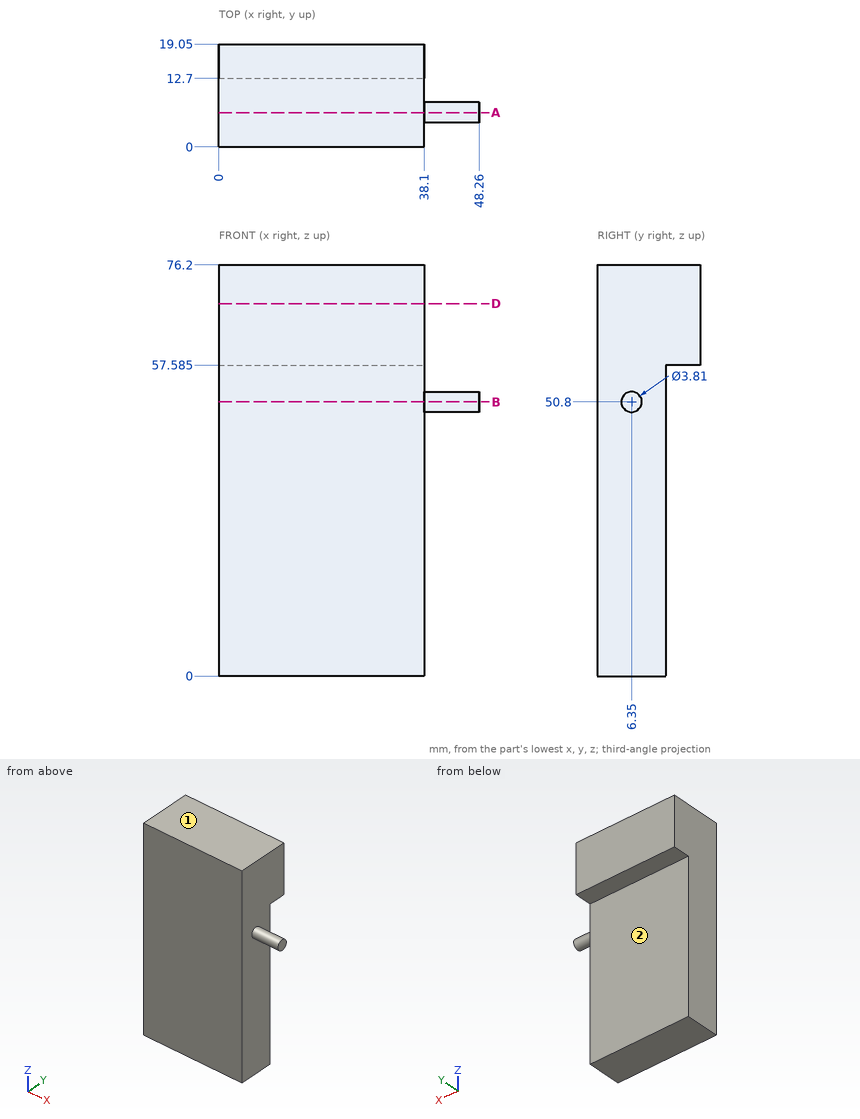
Geometry: see drawing. Coordinates: mm, zero at the bounding-box minimum. A direction names the side the tool comes from. Give positions to 0.01 mm unless a question says otherwise; leave off trailing zeros. Write each loop counter-clockwise with the first axis right and the second up, starting at its lowest first coordinate (ties: lowest second). Pieces come first, ordered by that corner, then holes. Notation, with made-up numbers: M 39.25,57 L 97.25,57 A5 ccw 97.25,66 Z; hole C 63.5,-10 d6. An arc over 180 degrees is marked long. Return JSON: item names as keys, results as strings. Group by question number.
1) First-contact query: pin 1 Ø3 at (x, y) = (23.5, 16) entering from -Z (1 decimal); pin 2 Ø5 at (y, z) = (10.5, 31.5) entering from +X; pin 3 Ø3 at (x, y) = (40.5, 7) entering from -Z (3 decimals). Flat tips, straight axial feed; report the tip coordinate or a pass-through.
2) Ray query, L1, parallel to Y at x = 21, z = 46.5; L2, parallel to X at y = 12, z = 63; L3, parallel to Z at x = 25.5, y = 14 (1 decimal). Return the intervals inside material, ascending.
3) Cut plane B-B, the plane z = 50.8. Output: boundary loops of the cut face in (x, y) (1 decimal).
4) Cut plane D-D, the plane z = 69. Output: boundary loops of the cut face in (x, y), then the cut area to 3 significant figures.
5) Cut plane A-A, the plane y = 6.35. Output: boundary loops of the cut face in (x, z) (1 decimal), then the cut area to 3 significant figures.
6) Set-up query: the marked faces 1 and 2. Return all of +Z, -Z, +X, -X, +Y, -Y with unobstructed straight access to the full face (end or side cutting, diameter ignored); none if empty.
Data:
{
 "1": {"pin 1": "stops at z = 57.6", "pin 2": "stops at x = 38.1", "pin 3": "stops at z = 48.895"},
 "2": {"L1": "y = 0 to 12.7", "L2": "x = 0 to 38.1", "L3": "z = 57.6 to 76.2"},
 "3": {"outline": "M 0,0 L 38.1,0 L 38.1,4.4 L 48.3,4.4 L 48.3,8.3 L 38.1,8.3 L 38.1,12.7 L 0,12.7 Z"},
 "4": {"outline": "M 0,0 L 38.1,0 L 38.1,19.05 L 0,19.05 Z", "area": "726 mm²"},
 "5": {"outline": "M 0,0 L 38.1,0 L 38.1,48.9 L 48.3,48.9 L 48.3,52.7 L 38.1,52.7 L 38.1,76.2 L 0,76.2 Z", "area": "2,940 mm²"},
 "6": {"face 1": "+Z, +X, -X, +Y, -Y", "face 2": "-Z, +X, -X, +Y"}
}
